from build123d import *

# Parameters (mm, degrees)
F0_W     = 36
F0_H     = 36
F0_R     = 1
F1_DEPTH = 1
F2_W     = 8.8
F2_H     = 8.8
F3_DEPTH = 6
F4_W     = 24.5
F4_H     = 5.5
F5_DEPTH = 2.3
F6_R     = 3.1
F7_DEPTH = 0.2


with BuildPart() as f1:
    # F0 (on Top) → F1 (new body)
    with BuildSketch(Plane.XY):
        Rectangle(F0_W, F0_H)
        with Locations((-16, -16)):
            Circle(F0_R, mode=Mode.SUBTRACT)
        with Locations((16, -16)):
            Circle(F0_R, mode=Mode.SUBTRACT)
        with Locations((-16, 16)):
            Circle(F0_R, mode=Mode.SUBTRACT)
        with Locations((16, 16)):
            Circle(F0_R, mode=Mode.SUBTRACT)
    extrude(amount=F1_DEPTH)

    # F2 (on face) → F3 (join)
    with BuildSketch(Plane.XY.offset(1)):
        Rectangle(F2_W, F2_H)
    extrude(amount=F3_DEPTH)

    # F4 (on face) → F5 (join)
    with BuildSketch(Plane(origin=(0, 0, 0), x_dir=(1, 0, 0), z_dir=(0, 0, -1))):
        with Locations((0, -15.25)):
            Rectangle(F4_W, F4_H)
    extrude(amount=F5_DEPTH)

    # F6 (on face) → F7 (join)
    with BuildSketch(Plane.XY.offset(7)):
        Circle(F6_R)
    extrude(amount=F7_DEPTH)


solid = f1.part
CAD build for the part. Positions are in the model's coordinates, mm. A direction names the side the tool comes from. Coordinates: 2 decimals unless noted, no trailing zeros. Write each loop counter-clockwise with the first axis right and the second up, starting at its lowest first coordinate (ties: lowest second). Pieces come first, ordered by that corner, then holes. Notation, with made-up numbers: M -34.5,72 L 14.5,72 A15 ccw 14.5,94 Z; hole C 11,-26.5 d1. An arc over 180 degrees is marked long. Return JSON: item names as keys, results as strings.
Item 1: Which spindle directions (+Z, -Z, +X, -X, +Y, -Y) get a long thin tool onto all of the face, cutting with end or side? Do faces 1 (the flat face through (4.4, 0, 4)), 2 (the flat face through (0, 4.4, 4)), 3 (the flat face through (-2, 3, 7)), 4 (the flat face through (-4.4, 0, 4)). Say none if no direction does.
Findings below:
{"face 1": "+Z, +X, +Y, -Y", "face 2": "+Z, +X, -X, +Y", "face 3": "+Z", "face 4": "+Z, -X, +Y, -Y"}
Item 2: Slice it at D-D, the plane x = 0. Write the cut outline in (y, z), and give its area (3 significant figures).
Findings below:
{"outline": "M -18,0 L 12.5,0 L 12.5,-2.3 L 18,-2.3 L 18,1 L 4.4,1 L 4.4,7 L 3.1,7 L 3.1,7.2 L -3.1,7.2 L -3.1,7 L -4.4,7 L -4.4,1 L -18,1 Z", "area": "103 mm2"}
Item 3: Probe line 1 (Y direction, x = 16, z = 0.5); line 2 (Z direction, x = -15, y = 1); line 3 (Y direction, x = 3, z = 5.25). List the from-to ranges inside material, lowest first. Write a range as from..to.
Findings below:
{"line 1": "y = -18..-17, -15..15, 17..18", "line 2": "z = 0..1", "line 3": "y = -4.4..4.4"}
Item 4: Slice it at C-C, the plane y = 0. Write the cut outline in (x, z).
Findings below:
{"outline": "M -18,0 L 18,0 L 18,1 L 4.4,1 L 4.4,7 L 3.1,7 L 3.1,7.2 L -3.1,7.2 L -3.1,7 L -4.4,7 L -4.4,1 L -18,1 Z"}
Item 5: Drop flat-ended pins along their axis: pin 1 Ø1.8 at (y, z) = (14, -1.5) entering from +X; pin 2 Ø3 at (x, z) = (1, 4.5) entering from -Y; pin 3 Ø5 at (x, y) = (-14, -0.5) entering from -Z; pin 4 Ø5 at (y, z) = (-4, 2) entering from -X. Give the stop position or say it passes through.
Findings below:
{"pin 1": "stops at x = 12.25", "pin 2": "stops at y = -4.4", "pin 3": "stops at z = 0", "pin 4": "stops at x = -18"}
Item 6: Slice it at A-A, the plane x = -16. Write the cut outline in (y, z).
Findings below:
{"outline": "M -18,0 L -17,0 L -17,1 L -18,1 Z; M -15,0 L 15,0 L 15,1 L -15,1 Z; M 17,0 L 18,0 L 18,1 L 17,1 Z"}
